Could you check a few things on this drawing? It's one solid part, dimensions in mm from its lowest x, y, z. Coordinates: 2 decimals unless noted, no trailing zeros. Order: outer loops, then holes, each group sorted by start corner. A loop starts at its lowest first (then second) coordinate and runs counter-clockwise, first axis right, second up. Notation, with made-up numbers: (86.25, -5.75) -> (115.25, -5.75) arc R5 ccw to (115.25, 2.25) -> close; hole circle Ø4 at (17, -29.5). An arc over 180 degrees is marked (long way). Use a Markdown table: item, result. Add a question column.
1. Suppose I cut it at A-A, the plane z = 6.5. List the corners of the cut face in (x, y) for me, then the cut area to 3 significant figures.
2. Suppose I cut it at D-D, the plane y = 1.5. List the corners of the cut face in (x, z) for me.
3. For pin 1 Ø8 at (x, z) = (12, 8) entering from -Y, with a flat end and sliding along its axis, tell me the tip position at first contact or that it passes through.
4. Suppose I cut it at C-C, the plane y = 0.45. List the corners of the cut face in (x, z) for me, then the cut area to 3 significant figures.
5. If I drill on line 1 along Z through (x, y) = (16.75, 1.05); line 2 along X through (y, z) = (0.55, 10.5); line 3 along Z through (x, y) = (16, 2.3), over which ranges is the centre line in solid material (lowest first)? Write a range as from..to.
6. Suppose I cut it at B-B, the plane x = 1.75. List the corners of the cut face in (y, z) for me, then the cut area to 3 significant figures.
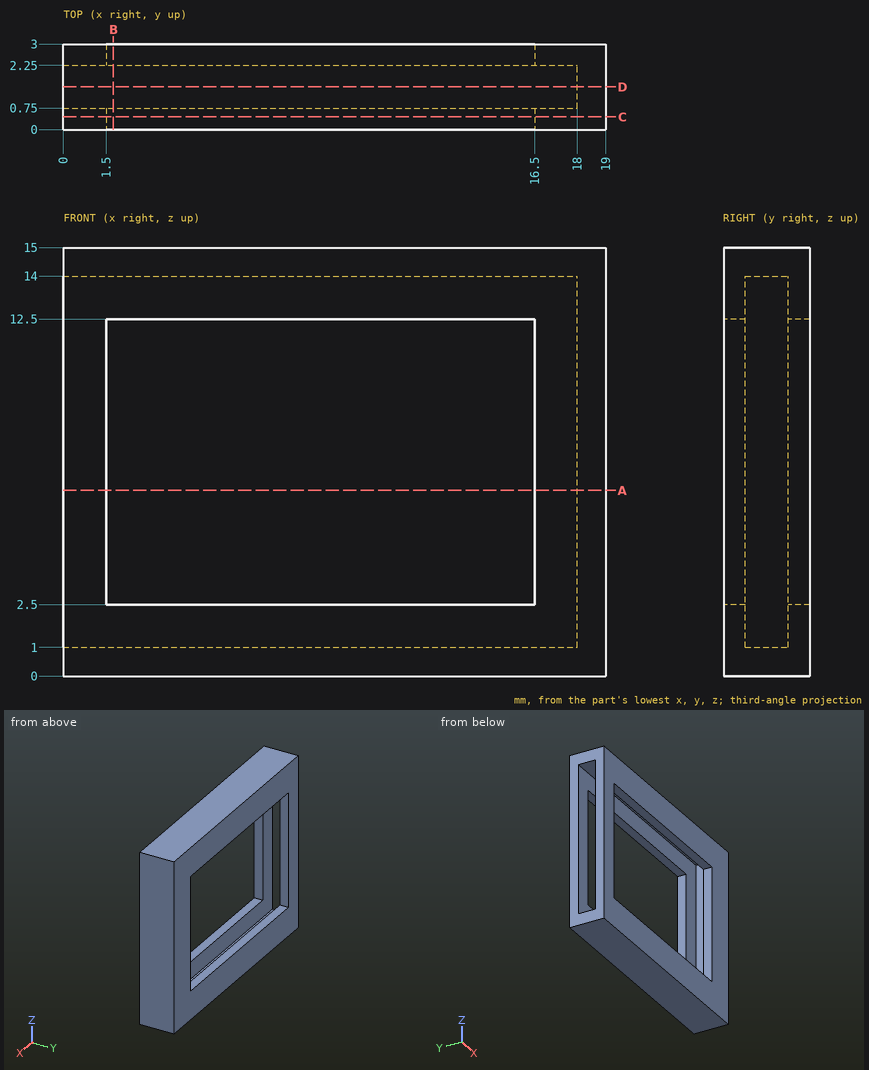
Worked out:
| question | item | result |
|---|---|---|
| 1 | outline | (0, 0) -> (1.5, 0) -> (1.5, 0.75) -> (0, 0.75) -> close; (0, 2.25) -> (1.5, 2.25) -> (1.5, 3) -> (0, 3) -> close; (16.5, 0) -> (19, 0) -> (19, 3) -> (16.5, 3) -> (16.5, 2.25) -> (18, 2.25) -> (18, 0.75) -> (16.5, 0.75) -> close |
| 1 | area | 7.50 mm² |
| 2 | outline | (0, 0) -> (19, 0) -> (19, 15) -> (0, 15) -> (0, 14) -> (18, 14) -> (18, 1) -> (0, 1) -> close |
| 3 | pin 1 | passes through |
| 4 | outline | (0, 0) -> (19, 0) -> (19, 15) -> (0, 15) -> close; hole (1.5, 2.5) -> (16.5, 2.5) -> (16.5, 12.5) -> (1.5, 12.5) -> close |
| 4 | area | 135 mm² |
| 5 | line 1 | z = 0..1, 14..15 |
| 5 | line 2 | x = 0..1.5, 16.5..19 |
| 5 | line 3 | z = 0..2.5, 12.5..15 |
| 6 | outline | (0, 0) -> (3, 0) -> (3, 2.5) -> (2.25, 2.5) -> (2.25, 1) -> (0.75, 1) -> (0.75, 2.5) -> (0, 2.5) -> close; (0, 12.5) -> (0.75, 12.5) -> (0.75, 14) -> (2.25, 14) -> (2.25, 12.5) -> (3, 12.5) -> (3, 15) -> (0, 15) -> close |
| 6 | area | 10.5 mm² |
